Read the model definition and answer for the solid it produces. Units are mm, in the model's axes. Face numbers are marked on the shaded views. A direction names the side the tool comes from. Coordinates: 2 decimals unless noted, no trailing zeros. Order: outer loops, then holes, each group sorted by start corner. A loop starts at its lowest first (then second) coordinate and runs counter-clockwise, first axis right, second up. Notation, with made-up numbers: M 65.25,-23.75 L 114.25,-23.75 A28 cw 114.25,5.25 Z; hole C 49.25,-26 d8. An arc over 180 degrees is marked long. Write each question's results on one line, items separated by ' | '.
```python
from build123d import *

# Parameters (mm, degrees)
BOSS_EXTRUDE1_DEPTH  = 5
SKETCH6_R            = 2
CUT_EXTRUDE3_DEPTH   = 53.239831546
SKETCH7_W            = 56
SKETCH7_H            = 6
BOSS_EXTRUDE2_DEPTH  = 28
SKETCH9_W            = 20
SKETCH9_H            = 28
BOSS_EXTRUDE3_DEPTH  = 2
SKETCH8_W            = 26
SKETCH8_H            = 33
BOSS_EXTRUDE4_DEPTH  = 2
BOSS_EXTRUDE5_START  = 28
SKETCH10_W           = 8
SKETCH10_H           = 20
SKETCH10_R           = 2
BOSS_EXTRUDE5_DEPTH  = 28
CUT_EXTRUDE4_DEPTH   = 20
SKETCH13_W           = 3.95
SKETCH13_H           = 4
CUT_EXTRUDE5_DEPTH   = 2
SKETCH14_W           = 60
SKETCH14_H           = 33
BOSS_EXTRUDE6_DEPTH  = 6
SKETCH15_R           = 2
BOSS_EXTRUDE7_DEPTH  = 20
SKETCH16_W           = 32
SKETCH16_H           = 33
BOSS_EXTRUDE8_DEPTH  = 12
SKETCH20_W           = 32
SKETCH20_H           = 33
BOSS_EXTRUDE9_DEPTH  = 5
SKETCH17_R           = 11.15
CUT_EXTRUDE6_DEPTH   = 7
CUT_EXTRUDE7_START   = -7
SKETCH19_R           = 11.15
CUT_EXTRUDE7_DEPTH   = 7
SKETCH21_R           = 8.5
CUT_EXTRUDE8_DEPTH   = 2
CUT_EXTRUDE10_START  = -28
SKETCH22_W           = 7
SKETCH22_H           = 8
CUT_EXTRUDE10_DEPTH  = 28
SKETCH25_W           = 8
SKETCH25_H           = 6
BOSS_EXTRUDE10_DEPTH = 28
CUT_EXTRUDE11_START  = -12
SKETCH26_R           = 2
CUT_EXTRUDE11_DEPTH  = 12
CUT_EXTRUDE12_START  = -2
SKETCH27_R           = 8.5
CUT_EXTRUDE12_DEPTH  = 2
CUT_EXTRUDE13_DEPTH  = 0.2
CUT_EXTRUDE14_DEPTH  = 0.2


with BuildPart() as part:
    # Sketch2 → Boss-Extrude1 (new body)
    with BuildSketch(Plane(origin=(0, 0, 0), x_dir=(1, 0, 0), z_dir=(0, 1, 0))):
        Polygon((0, 0), (0, 20), (-8, 20), (-8, -6), (48, -6), (48, 20), (40, 20), (40, 0), align=None)
    extrude(amount=BOSS_EXTRUDE1_DEPTH)

    # Sketch6 → Cut-Extrude3 (cut, through all)
    with BuildSketch(Plane.XZ):
        with Locations(Location((43.95, -5, 0), (0, 0, 270))):
            Circle(SKETCH6_R)
        with Locations(Location((43.95, -15, 0), (0, 0, 270))):
            Circle(SKETCH6_R)
        with Locations(Location((-3.95, -5, 0), (0, 0, 270))):
            Circle(SKETCH6_R)
        with Locations(Location((-3.95, -15, 0), (0, 0, 270))):
            Circle(SKETCH6_R)
    extrude(amount=-CUT_EXTRUDE3_DEPTH, mode=Mode.SUBTRACT)

    # Sketch7 → Boss-Extrude2 (add)
    with BuildSketch(Plane.XZ):
        with Locations((20, 3)):
            Rectangle(SKETCH7_W, SKETCH7_H)
    extrude(amount=BOSS_EXTRUDE2_DEPTH)

    # Sketch9 → Boss-Extrude3 (add)
    with BuildSketch(Plane.ZY.offset(8)):
        Polygon((-20, 5), (-20, 0), (0, 0), (0, -28), (6, -28), (6, 5), align=None)
        with Locations((-10, -14)):
            Rectangle(SKETCH9_W, SKETCH9_H)
    extrude(amount=BOSS_EXTRUDE3_DEPTH)

    # Sketch8 → Boss-Extrude4 (add)
    with BuildSketch(Plane(origin=(48, 0, 0), x_dir=(0, 0, -1), z_dir=(1, 0, 0))):
        with Locations((7, -11.5)):
            Rectangle(SKETCH8_W, SKETCH8_H)
    extrude(amount=BOSS_EXTRUDE4_DEPTH)

    # Sketch10 → Boss-Extrude5 (add)
    with BuildSketch(Plane.XZ.offset(BOSS_EXTRUDE5_START)):
        with Locations((-4, -10)):
            Rectangle(SKETCH10_W, SKETCH10_H)
        with Locations(Location((-3.95, -5, 0), (0, 0, 270))):
            Circle(SKETCH10_R, mode=Mode.SUBTRACT)
        with Locations(Location((-3.95, -15, 0), (0, 0, 270))):
            Circle(SKETCH10_R, mode=Mode.SUBTRACT)
    extrude(amount=-BOSS_EXTRUDE5_DEPTH)

    # Sketch12 → Cut-Extrude4 (cut)
    with BuildSketch(Plane(origin=(0, 0, -20), x_dir=(-1, 0, 0), z_dir=(0, 0, -1))):
        Polygon((-40, 5), (-40, 2.5), (-40.83785019, 5), align=None)
        Polygon((0, -6.167201623), (1.617522403, 5), (0, 5), align=None)
    extrude(amount=-CUT_EXTRUDE4_DEPTH, mode=Mode.SUBTRACT)

    # Sketch13 → Cut-Extrude5 (cut)
    with BuildSketch(Plane(origin=(0, 5, 0), x_dir=(1, 0, 0), z_dir=(0, 1, 0))):
        with Locations((-1.975, 5)):
            Rectangle(SKETCH13_W, SKETCH13_H)
        with Locations((-1.975, 15)):
            Rectangle(SKETCH13_W, SKETCH13_H)
    extrude(amount=-CUT_EXTRUDE5_DEPTH, mode=Mode.SUBTRACT)

    # Sketch14 → Boss-Extrude6 (add)
    with BuildSketch(Plane(origin=(0, 0, -20), x_dir=(-1, 0, 0), z_dir=(0, 0, -1))):
        with Locations((-20, -11.5)):
            Rectangle(SKETCH14_W, SKETCH14_H)
    extrude(amount=BOSS_EXTRUDE6_DEPTH)

    # Sketch15 → Boss-Extrude7 (add)
    with BuildSketch(Plane.XZ.offset(28)):
        with Locations(Location((-3.95, -5, 0), (0, 0, 270))):
            Circle(SKETCH15_R)
        with Locations(Location((-3.95, -15, 0), (0, 0, 270))):
            Circle(SKETCH15_R)
    extrude(amount=-BOSS_EXTRUDE7_DEPTH)

    # Sketch16 → Boss-Extrude8 (add)
    with BuildSketch(Plane(origin=(50, 0, 0), x_dir=(0, 0, -1), z_dir=(1, 0, 0))):
        with Locations((10, -11.5)):
            Rectangle(SKETCH16_W, SKETCH16_H)
    extrude(amount=BOSS_EXTRUDE8_DEPTH)

    # Sketch20 → Boss-Extrude9 (add)
    with BuildSketch(Plane.ZY.offset(10)):
        with Locations((-10, -11.5)):
            Rectangle(SKETCH20_W, SKETCH20_H)
    extrude(amount=BOSS_EXTRUDE9_DEPTH)

    # Sketch17 → Cut-Extrude6 (cut)
    with BuildSketch(Plane(origin=(62, 0, 0), x_dir=(0, 0, -1), z_dir=(1, 0, 0))):
        with Locations((10, -12)):
            Circle(SKETCH17_R)
    extrude(amount=-CUT_EXTRUDE6_DEPTH, mode=Mode.SUBTRACT)

    # Sketch19 → Cut-Extrude7 (cut)
    with BuildSketch(Plane.ZY.offset(15).offset(CUT_EXTRUDE7_START)):
        with Locations(Location((-10, -12, 0), (0, 0, 180))):
            Circle(SKETCH19_R)
    extrude(amount=CUT_EXTRUDE7_DEPTH, mode=Mode.SUBTRACT)

    # Sketch21 → Cut-Extrude8 (cut)
    with BuildSketch(Plane(origin=(55, 0, 0), x_dir=(0, 0, -1), z_dir=(1, 0, 0))):
        with Locations((10, -12)):
            Circle(SKETCH21_R)
    extrude(amount=-CUT_EXTRUDE8_DEPTH, mode=Mode.SUBTRACT)

    # Sketch22 → Cut-Extrude10 (cut)
    with BuildSketch(Plane.XZ.offset(28).offset(CUT_EXTRUDE10_START)):
        with Locations((51.5, -10)):
            Rectangle(SKETCH22_W, SKETCH22_H)
    extrude(amount=CUT_EXTRUDE10_DEPTH, mode=Mode.SUBTRACT)

    # Sketch25 → Boss-Extrude10 (add)
    with BuildSketch(Plane.XZ):
        with Locations((44, -3)):
            Rectangle(SKETCH25_W, SKETCH25_H)
        with Locations((44, -17)):
            Rectangle(SKETCH25_W, SKETCH25_H)
    extrude(amount=BOSS_EXTRUDE10_DEPTH)

    # Sketch26 → Cut-Extrude11 (cut)
    with BuildSketch(Plane(origin=(0, 5, 0), x_dir=(1, 0, 0), z_dir=(0, 1, 0)).offset(CUT_EXTRUDE11_START)):
        with Locations(Location((43.95, 5, 0), (0, 0, 90))):
            Circle(SKETCH26_R)
        with Locations(Location((43.95, 15, 0), (0, 0, 90))):
            Circle(SKETCH26_R)
    extrude(amount=CUT_EXTRUDE11_DEPTH, mode=Mode.SUBTRACT)

    # Sketch27 → Cut-Extrude12 (cut)
    with BuildSketch(Plane.ZY.offset(8).offset(CUT_EXTRUDE12_START)):
        with Locations((-10, -12)):
            Circle(SKETCH27_R)
    extrude(amount=CUT_EXTRUDE12_DEPTH, mode=Mode.SUBTRACT)

    # Sketch28 → Cut-Extrude13 (cut)
    with BuildSketch(Plane(origin=(0, 0, 0), x_dir=(-1, 0, 0), z_dir=(0, 0, -1))):
        Polygon((-40, 2.5), (-40, -28), (0, -28), (0, -6.167201623), (1.617522403, 5), (-40.83785019, 5), align=None)
    extrude(amount=-CUT_EXTRUDE13_DEPTH, mode=Mode.SUBTRACT)

    # Sketch29 → Cut-Extrude14 (cut)
    with BuildSketch(Plane.XY.offset(-20)):
        Polygon((0, -28), (40, -28), (40, 2.5), (40.83785019, 5), (-1.617522403, 5), (0, -6.167201623), align=None)
    extrude(amount=-CUT_EXTRUDE14_DEPTH, mode=Mode.SUBTRACT)


solid = part.part
```
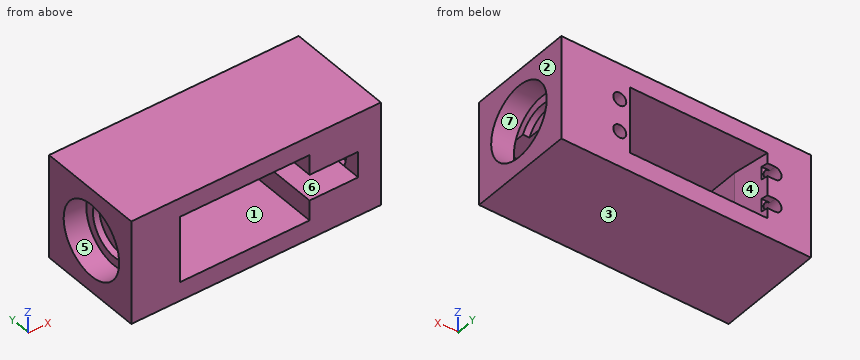
(1) Straight lines are drawn through the part: line 1 (Z direction, x = 6.5, y = -4); line 2 (X direction, y = -0.5, z = -5); line 3 (X direction, y = 0, z = -5). For each, find the intervals that lie inside material, in ascending order.
Conclusion:
line 1: -26 to -20.2, 0.2 to 6 | line 2: -15 to -5.95, -1.95 to -0.82, 40 to 41.95, 45.95 to 62 | line 3: -15 to -5.95, -1.95 to -0.89, 40 to 41.95, 45.95 to 62
(2) For the marked faces 4, 5, 6 and 7, determine the directions among +Z, -Z, +X, -X, +Y, -Y from which every point of the face is accessible in a straight line to the end or side of a thin tool.
Conclusion:
face 4: +Y | face 5: -X | face 6: -Y | face 7: +X
(3) The part is cut by section C-C, the plane x = 24. Write down the section's boundary in (y, z), then the cut area to 3 significant figures.
Conclusion:
outline: M -28,-26 L 5,-26 L 5,-20.2 L -28,-20.2 Z; M -28,0.2 L 5,0.2 L 5,6 L -28,6 Z | area: 383 mm²
(4) The part is cut by section A-A, the plane x = 43.95. Write down the section's boundary in (y, z), then the cut area to 3 significant figures.
Conclusion:
outline: M -28,-26 L 5,-26 L 5,-17 L -7,-17 L -7,-14 L -28,-14 Z; M -28,-6 L -7,-6 L -7,-3 L 5,-3 L 5,6 L -28,6 Z; M 0,-13 L 5,-13 L 5,-7 L 0,-7 Z | area: 750 mm²
(5) The mould has two halves that part along Z. Classify the marked faces 1, 2 and 3: pulls with the +Z half, pulls with the -Z half, needs draft (parallel to the pull), parting line crosses it, or undercut.
Conclusion:
face 1: undercut | face 2: needs draft | face 3: pulls with the -Z half
(6) The part is cut by section B-B, the plane z = -10. Write down the section's boundary in (x, y), then the cut area to 3 significant figures.
Conclusion:
outline: M -15,-28 L 0,-28 L 0,-6.17 L -1.62,5 L -15,5 L -15,-0.85 L -8,-0.85 L -8,-3.5 L -6,-3.5 L -6,-20.5 L -8,-20.5 L -8,-23.15 L -15,-23.15 Z; M 40,0 L 55,0 L 55,-0.85 L 62,-0.85 L 62,5 L 40.84,5 L 40,2.5 Z; M 55,-28 L 62,-28 L 62,-23.15 L 55,-23.15 Z | area: 445 mm²
(7) Given pin 1 (0.9 mm diameter, centred on x = 43.5, z = -4, fed in from +Y); pin 2 (8.5 mm diameter, centred on y = -16, z = -10, fed in from -X); pin 3 (5 mm diameter, centred on y = -11, z = -10.5, fed in from +X), each flat-ended and moving along its own axis, determine where each tip first touches the part or whether it passes through.
Conclusion:
pin 1: y = -7 | pin 2: x = -6 | pin 3: x = 0
